```python
from build123d import *

# Parameters (mm, degrees)
F0_R     = 23.8125
F1_DEPTH = 19.05
F0_R_2   = 12.7
F2_DEPTH = 6.35
F3_SIZE  = 0.508
F4_R     = 2.54
F5_DEPTH = 25.4
F6_R     = 3.175


with BuildPart() as f1:
    # F0 (on Right) → F1 (new body)
    with BuildSketch(Plane.YZ):
        with BuildLine():
            Line((-38.1, -76.2), (38.1, -76.2))
            Line((38.1, -76.2), (38.1, 0))
            ThreePointArc((38.1, 0), (0, 38.1), (-38.1, 0))
            Line((-38.1, 0), (-38.1, -76.2))
        make_face()
        Circle(F0_R, mode=Mode.SUBTRACT)
    extrude(amount=F1_DEPTH)

    # F0 (on Right) → F2 (join)
    with BuildSketch(Plane.YZ):
        Circle(F0_R)
        Circle(F0_R_2, mode=Mode.SUBTRACT)
    extrude(amount=F2_DEPTH)

    # F3
    f3_edges = [f1.edges().sort_by_distance(p)[0] for p in [
        (0, -12.7, 0),
        (19.05, -23.8125, 0),
        (6.35, -12.7, 0),
    ]]
    chamfer(f3_edges, length=F3_SIZE)

    # F4 (on face) → F5 (cut)
    with BuildSketch(Plane(origin=(0, 0, -76.2), x_dir=(1, 0, 0), z_dir=(0, 0, -1))):
        with Locations((9.525, 25.4)):
            Circle(F4_R)
        with Locations((9.525, -25.4)):
            Circle(F4_R)
    extrude(amount=-F5_DEPTH, mode=Mode.SUBTRACT)

    # F6
    f6_edges = [f1.edges().sort_by_distance(p)[0] for p in [
        (19.05, -38.1, -38.1),
        (0, -38.1, -38.1),
    ]]
    fillet(f6_edges, radius=F6_R)


solid = f1.part
```
Geometry check sheet. Reference: the model listing, model coordinates, mm. A direction names the side the tool comes from. Give positions to 0.01 mm unless a question says otherwise; leave off trailing zeros. Loops run counter-clockwise (first coordinate to the right, second up) from the corner with the lowest first, then second, coordinate; pieces in that order, holes last. Notation, with made-up numbers: M -21,59.5 L 20,59.5 A36 ccw 20,95.5 Z; hole C 13,4.5 d5. An arc over 180 degrees is marked long. Write item = value, one per line. Start each with the question number.
1. Section check C-C, the plane x = 9.5. Enter the section's corners in (y, z) (1 decimal), plus the area to 3 significant figures.
2. Section check B-B, the plane z = -53. Enter the section's corners in (x, y) (3 decimals).
3. Tool access check on faces 5 (the face through (9.194, -27.918, -63.678)), 6 (the face through (19.05, 0, -32)). Record the directions out of +Z, -Z, +X, -X, +Y, -Y that give a thin tool (end or side, any length) a straight path to the whole face; none if there is none.
4. Go/stop test with flat-tipped pins: P1, Ø1.5, axis at x = 17, y = 6, coming from the +Z side; P2, Ø6, axis at x = 9, y = -22, coming from the +Z side; P3, Ø1.5, axis at x = 9.5, y = -25.5, coming from the -Z side. Record where each tip stops, or that it passes through.
5. Draft check along Z on faces 1 (the face through (3.14, -2.75, -12.4)), 2 (the face through (9, -38.1, -38)), 3 (the face through (9.44, 0.84, 38.09)), 4 (the face through (12.361, -18.897, -14.49)). Enter one of: +Z half, -Z half, draft (parallel to the pull), parting line (faces both ways), or undercut.
6. Thickness scan on probe 1 along Y at (x, z) = (8, -67.5); probe 2 along Y at (x, z) = (11.75, -71); probe 3 along Z at (x, y) = (5.75, 2). Record the ranges inside material, lowest first.
7. Section check D-D, the plane x = 17. Enter the section's corners in (y, z) (1 decimal).
Values follow:
q1.outline = M -38.1,-76.2 L -27.9,-76.2 L -27.9,-50.8 L -22.9,-50.8 L -22.9,-76.2 L 22.9,-76.2 L 22.9,-50.8 L 27.9,-50.8 L 27.9,-76.2 L 38.1,-76.2 L 38.1,0 A38.1 ccw -38.1,0 Z; hole C 0,0 d47.6
q1.area = 6,050 mm^2
q2.outline = M 0,-34.925 A3.175 ccw 3.175,-38.1 L 15.875,-38.1 A3.175 ccw 19.05,-34.925 L 19.05,34.925 A3.175 ccw 15.875,38.1 L 3.175,38.1 A3.175 ccw 0,34.925 Z; hole C 9.525,-25.4 d5.08; hole C 9.525,25.4 d5.08
q3.face_5 = -Z
q3.face_6 = +Z, -Z, +X, +Y, -Y
q4.P1 = 37.65
q4.P2 = 33.02
q4.P3 = -50.8
q5.face_1 = undercut
q5.face_2 = draft
q5.face_3 = +Z half
q5.face_4 = undercut
q6.probe_1 = -38.1 to -27.43, -23.37 to 23.37, 27.43 to 38.1
q6.probe_2 = -38.1 to -26.63, -24.17 to 24.17, 26.63 to 38.1
q6.probe_3 = -76.2 to -12.54, 12.54 to 38.05
q7.outline = M -37.9,-76.2 L 37.9,-76.2 L 37.9,0 A37.9 ccw -37.9,0 Z; hole C 0,0 d47.6
